Geometry check sheet. Reference: the model listing, model coordinates, mm. Face numbers are marked on the shaded views. A direction names the side the tool comes from. Coordinates: 2 decimals unless noted, no trailing zeros. Write each loop counter-clockwise with the first axis right and the second up, starting at its lowest first coordinate (ties: lowest second). Pieces come first, ordered by that corner, then holes. Notation, with made-up numbers: (-16.75, 38) -> (-11.75, 38) arc R24 ccw to (-11.75, 56) -> close; hole circle Ø8 at (14, 26). An arc over 180 degrees is marked (long way). Use a Markdown table: item, result.
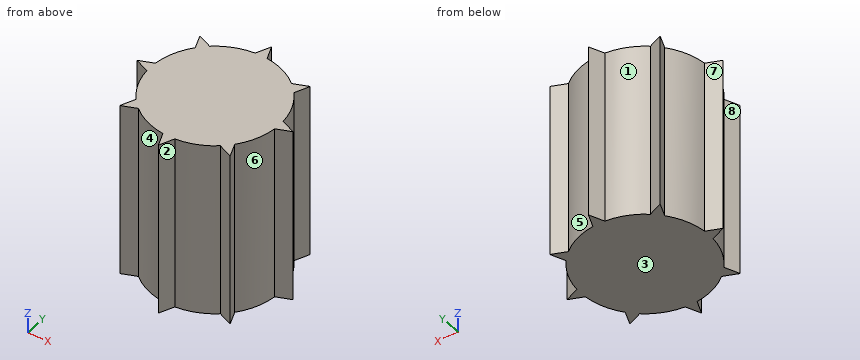
```python
from build123d import *

# Parameters (mm, degrees)
SALIENTE_EXTRUIR1_DEPTH = 85


with BuildPart() as part:
    # Croquis1 → Saliente-Extruir1 (new body)
    with BuildSketch(Plane.XY):
        with BuildLine():
            Line((-2.940383589, 30.958198867), (0, 37.891714368))
            Line((0, 37.891714368), (2.798692732, 30.971329512))
            ThreePointArc((2.798692732, 30.971329512), (11.834742576, 28.757517294), (19.811587178, 23.969917527))
            Line((19.811587178, 23.969917527), (26.79348818, 26.79348818))
            Line((26.79348818, 26.79348818), (23.879011729, 19.921062511))
            ThreePointArc((23.879011729, 19.921062511), (28.703062218, 11.96620876), (30.958198867, 2.940383589))
            Line((30.958198867, 2.940383589), (37.891714368, 0))
            Line((37.891714368, 0), (30.971329512, -2.798692732))
            ThreePointArc((30.971329512, -2.798692732), (28.757517294, -11.834742576), (23.969917527, -19.811587178))
            Line((23.969917527, -19.811587178), (26.79348818, -26.79348818))
            Line((26.79348818, -26.79348818), (19.921062511, -23.879011729))
            ThreePointArc((19.921062511, -23.879011729), (11.96620876, -28.703062218), (2.940383589, -30.958198867))
            Line((2.940383589, -30.958198867), (0, -37.891714368))
            Line((0, -37.891714368), (-2.798692732, -30.971329512))
            ThreePointArc((-2.798692732, -30.971329512), (-11.834742576, -28.757517294), (-19.811587178, -23.969917527))
            Line((-19.811587178, -23.969917527), (-26.79348818, -26.79348818))
            Line((-26.79348818, -26.79348818), (-23.879011729, -19.921062511))
            ThreePointArc((-23.879011729, -19.921062511), (-28.703062218, -11.96620876), (-30.958198867, -2.940383589))
            Line((-30.958198867, -2.940383589), (-37.891714368, 0))
            Line((-37.891714368, 0), (-30.971329512, 2.798692732))
            ThreePointArc((-30.971329512, 2.798692732), (-28.757517294, 11.834742576), (-23.969917527, 19.811587178))
            Line((-23.969917527, 19.811587178), (-26.79348818, 26.79348818))
            Line((-26.79348818, 26.79348818), (-19.921062511, 23.879011729))
            ThreePointArc((-19.921062511, 23.879011729), (-11.96620876, 28.703062218), (-2.940383589, 30.958198867))
        make_face()
    extrude(amount=SALIENTE_EXTRUIR1_DEPTH)


solid = part.part
```
Item 1: Section check B-B on y = -21.5. Record the boundary of the cut face in (x, z).
Answer block:
| item | result |
|---|---|
| outline | (-24.55, 0) -> (24.65, 0) -> (24.65, 85) -> (-24.55, 85) -> close |
Item 2: Section check A-A on z = 38.5. Record the boundary of the cut face in (x, y).
Answer block:
| item | result |
|---|---|
| outline | (-37.89, 0) -> (-30.96, -2.94) arc R31.1 ccw to (-23.88, -19.92) -> (-26.79, -26.79) -> (-19.81, -23.97) arc R31.1 ccw to (-2.8, -30.97) -> (0, -37.89) -> (2.94, -30.96) arc R31.1 ccw to (19.92, -23.88) -> (26.79, -26.79) -> (23.97, -19.81) arc R31.1 ccw to (30.97, -2.8) -> (37.89, 0) -> (30.96, 2.94) arc R31.1 ccw to (23.88, 19.92) -> (26.79, 26.79) -> (19.81, 23.97) arc R31.1 ccw to (2.8, 30.97) -> (0, 37.89) -> (-2.94, 30.96) arc R31.1 ccw to (-19.92, 23.88) -> (-26.79, 26.79) -> (-23.97, 19.81) arc R31.1 ccw to (-30.97, 2.8) -> close |
Item 3: Section check C-C on x = 18.5. Record the boundary of the cut face in (y, z), then the cut area to 3 significant figures.
Answer block:
| item | result |
|---|---|
| outline | (-25, 0) -> (25, 0) -> (25, 85) -> (-25, 85) -> close |
| area | 4,250 mm^2 |
Item 4: Thickness scan on L1, parallel to Y at x = 26.5, z = 61.5; L2, parallel to Y at x = 26, z = 68; L3, parallel to X at y = -31, z = 78. Record the ranges inside material, lowest first. Write a range as [from, to].
Answer block:
| item | result |
|---|---|
| L1 | y = [-26.67, -26.07], [-16.27, 16.27], [26.1, 26.67] |
| L2 | y = [-26.46, -24.83], [-17.06, 17.06], [24.92, 26.47] |
| L3 | x = [-2.79, 2.92] |
Item 5: Mould release check, pull along X, two halves, no side actions. Record for the marked faces 1, 2 and 3: +X half, -X half, draft (parallel to the pull), parting line (faces both ways), or undercut.
Answer block:
| item | result |
|---|---|
| face 1 | undercut |
| face 2 | +X half |
| face 3 | draft |
Item 6: Depth check by flat-ended pin: P1, Ø1.5, axis at x = -6, z = 64.5, coming from the -Y side; P2, Ø3, axis at x = -14, z = 70.5, coming from the -Y side; P3, Ø6, axis at x = -6.5, y = -4, coming from the -Z side; P4, Ø2, axis at x = 6, z = 73.5, coming from the +Y side. Enter the tip coordinate at first touch or a pass-through.
Answer block:
| item | result |
|---|---|
| P1 | stops at y = -30.65 |
| P2 | stops at y = -28.47 |
| P3 | stops at z = 0 |
| P4 | stops at y = 30.69 |
Item 7: Tool access check on the marked faces 4, 5, 6, 7 and 8. Record the directions out of +Z, -Z, +X, -X, +Y, -Y that give a thin tool (end or side, any length) a straight path to the whole face; none if there is none.
Answer block:
| item | result |
|---|---|
| face 4 | +Z, -Z, -Y |
| face 5 | +Z, -Z, +Y |
| face 6 | +Z, -Z, +X |
| face 7 | +Z, -Z, -X, +Y |
| face 8 | +Z, -Z, -X |
